Autodesk Inventor part; units mm, degrees
ref_plane "YZ Plane" through (0, 0, 0) normal (1, 0, 0) x (0, 1, 0)
ref_plane "XZ Plane" through (0, 0, 0) normal (0, 1, 0) x (-1, 0, 0)
ref_plane "XY Plane" through (0, 0, 0) normal (0, 0, 1) x (1, 0, 0)
sketch "Эскиз1" plane through (0, 0, 0) normal (0, 1, 0) x (-1, 0, 0)
  line L0 (0, 0) -> (60, 0)
  line L1 (60, 0) -> (60, -45)
  line L2 (60, -45) -> (0, -45)
  line L3 (0, -45) -> (0, 0)
  line L4 (0, -22.5) -> (0, 0)
  line L5 (0, 0) -> (0, -10)
  line L6 (0, -10) -> (35, -10)
  line L7 (35, -10) -> (35, -35)
  line L8 (35, -35) -> (0, -35)
  line L9 (35, -22.5) -> (45, -22.5)
  dimension "d0" = 60
  dimension "d1" = 45
  dimension "d3" = 10
  dimension "d4" = 35
  dimension "d5" = 25
  dimension "d6" = 10
extrude "Выдавливание1" add sketch "Эскиз1" along normal blind 10 contours L0 L1 L2 L3 L8 L7 L6
sketch "Эскиз3" plane through (0, 0, -35) normal (1, 0, 0) x (0, 0, -1)
  line L0 (10, 10) -> (-35, 10)
  line L1 (10, 10) -> (-35, 10)
  line L2 (-35, 10) -> (-35, -26)
  line L3 (-35, -26) -> (10, -26)
  line L4 (10, -26) -> (10, 10)
  point P0 (-35, 0)
  dimension "d13" = 45
  dimension "d14" = 36
extrude "Выдавливание3" add sketch "Эскиз3" along normal blind 5
sketch "Эскиз4" plane through (0, -26, -45) normal (0, -1, 0) x (1, 0, 0)
  line L0 (-60, 0) -> (0, 0)
  line L1 (0, 0) -> (0, 45)
  line L2 (0, 45) -> (-60, 45)
  line L3 (-60, 45) -> (-60, 0)
  line L4 (0, 35) -> (-35, 35)
  line L5 (-35, 10) -> (0, 10)
  line L6 (0, 10) -> (0, 35)
  line L7 (0, 35) -> (-35, 35)
  line L8 (-35, 35) -> (-35, 10)
extrude "Выдавливание4" add sketch "Эскиз4" against normal blind 10 contours L3 L2 L1 L4 L8 L5 L0
sketch "Эскиз5" plane through (0, 0, 0) normal (0, -1, 0) x (1, 0, 0)
  line L0 (-35, -10) -> (-35, -35)
  line L1 (-35, -22.5) -> (-45, -22.5)
  circle A0 centre (-45, -22.5) radius 5
  point P0 (0, 0)
  dimension "d19" = 10
  dimension "d20" = 10
extrude "Выдавливание5" cut sketch "Эскиз5" along normal blind 24 and the other way blind 6
sketch "Эскиз6" plane through (5, -26, -45) normal (0, -1, 0) x (1, 0, 0)
  line L0 (0, 0) -> (0, 45)
  line L1 (-65, 0) -> (0, 0)
  line L2 (0, 45) -> (-5, 45)
  line L3 (-5, 45) -> (-5, 0)
  line L4 (-5, 0) -> (0, 0)
  line L5 (0, 0) -> (0, 45)
extrude "Выдавливание6" add sketch "Эскиз6" along normal blind 50
sketch "Эскиз7" plane through (5, -76, -45) normal (0, -1, 0) x (1, 0, 0)
  line L0 (-65, 45) -> (0, 45)
  line L1 (0, 45) -> (-65, 45)
  line L2 (-65, 45) -> (-65, 0)
  line L3 (-65, 0) -> (0, 0)
  line L4 (0, 0) -> (0, 45)
  line L5 (-5, 10) -> (-5, 35)
  line L6 (-5, 22.5) -> (-15, 22.5)
  line L7 (-15, 22.5) -> (-17.5, 22.5)
  circle A0 centre (-17.5, 22.5) radius 2.5
  point P0 (-5, 45)
  dimension "d27" = 10
  dimension "d28" = 2.5
extrude "Выдавливание7" add sketch "Эскиз7" along normal blind 1
sketch "Эскиз8" plane through (0, 0, -35) normal (-1, 0, 0) x (0, 0, 1)
  line L0 (0, 0) -> (-10, 0)
  line L1 (-10, -16) -> (35, -16)
  line L2 (-10, 0) -> (-5, 0)
  line L3 (-5, 0) -> (-5, -16)
  line L4 (-5, -16) -> (-10, -16)
  line L5 (-10, -16) -> (-10, 0)
  line L6 (-10, 0) -> (35, 0)
  line L7 (35, -16) -> (30, -16)
  line L8 (30, -16) -> (30, 0)
  line L9 (30, 0) -> (35, 0)
  line L10 (35, 0) -> (35, -16)
  point P0 (25, -16)
  point P1 (-5, 0)
  dimension "d31" = 5
  dimension "d34" = 5
extrude "Выдавливание8" add sketch "Эскиз8" along normal blind 10 contours L3 L1 L5 L0 | L6 L10 L1 L8
properties part number "Стенка"
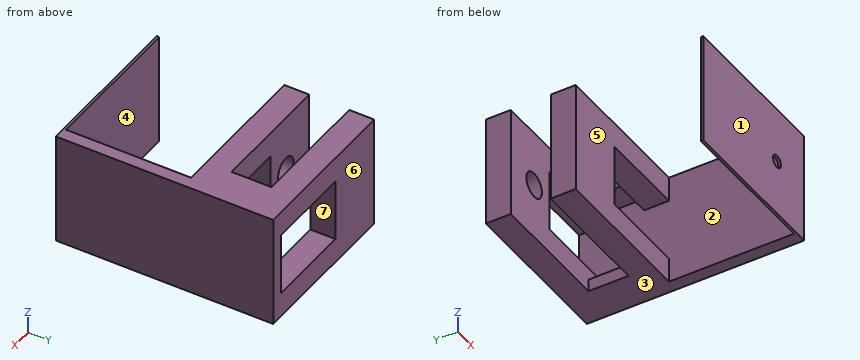
Design review of the part built by this model. Coordinates are the model's own, in mm. Face numbers are marked on the shaded views. A direction names the side the tool comes from. Give positions to 0.01 mm unless a question says otherwise; leave off trailing zeros. Order: outer loops, then holes, each group sorted by start corner. A loop starts at its lowest first (then second) coordinate and runs counter-clockwise, first axis right, second up. Notation, with made-up numbers: (-39.5, -37) - (-27.5, -37) arc R23 ccw to (-27.5, -24) - close; hole circle Ø6 at (-12.5, -38). An arc over 180 degrees is marked (long way). Use a Markdown table: item, result. Add a question column.
(1) Add section B-B on z = -22.5. Give the boundary of the cut face in (x, y), then the cut area to 3 significant figures.
(2) Add section D-D on z = -31.5. Give the boundary of the cut face in (x, y).
(3) Add section C-C on x = -12.5. Give the boundary of the cut face in (y, z).
(4) Mouldability with a two-part tool opening along Y and no side actions: class the marked faces 1, 2, 3 and 4 as +Y half, -Y half, draft (parallel to the pull), parting line (faces both ways), or undercut.
(5) Machinability: for the marked faces 5, 6 and 7, which of the approach directions +Z, -Z, +X, -X, +Y, -Y give a long, thin tool a straight path to every point of the face, cutting with its end or side? Answer none if there is none.
(6) Wall thickness on probe 1 along Y at (x, z) = (-49, -15.5); probe 2 along Z at (x, y) = (-8, -17); probe 3 along X at (y, z) = (-13.5, -18.5): over which ranges is each line inside the solid? List them lowest first. Write a range as [from, to].
(7) Clearance check with flat-ended pins moving along their axes: P1, Ø13.5, axis at x = -32, z = -24, coming from the +Y side; P2, Ø5.5, axis at y = -8.5, z = -1.5, coming from the -X side; P3, Ø4, axis at x = -12.5, z = -22.5, coming from the +Y side; P4, Ø5, axis at x = -15.5, z = -13, coming from the +Y side. State where each tip first meets the part, or that it passes through.
(8) Add section A-A on x = -27. Give the boundary of the cut face in (y, z), then the cut area to 3 significant figures.
Report:
| question | item | result |
|---|---|---|
| 1 | outline | (-60, -77) - (-15, -77) - (-15, -76) - (-60, -76) - close; (-60, -26) - (-35, -26) - (-35, -16) - (-40, -16) - (-40, -24) - (-50, -24) - (-50, -16) - (-60, -16) - close; (-60, 0) - (-50, 0) - (-50, 6) - (-40, 6) - (-40, 0) - (-35, 0) - (-35, 10) - (-60, 10) - close; (-10, -77) - (5, -77) - (5, 10) - (0, 10) - (0, -76) - (-10, -76) - close |
| 1 | area | 850 mm² |
| 2 | outline | (-60, -77) - (5, -77) - (5, 10) - (0, 10) - (0, -76) - (-60, -76) - close; (-60, -26) - (-35, -26) - (-35, -16) - (-60, -16) - close; (-60, 0) - (-35, 0) - (-35, 10) - (-60, 10) - close |
| 3 | outline | (-77, -45) - (-76, -45) - (-76, -25) - (-77, -25) - close; (-77, -20) - (-76, -20) - (-76, 0) - (-77, 0) - close; (-26, -45) - (-16, -45) - (-16, -35) - (-26, -35) - close; (-26, -10) - (-16, -10) - (-16, 0) - (-26, 0) - close; (0, -45) - (10, -45) - (10, -35) - (0, -35) - close; (0, -10) - (10, -10) - (10, 0) - (0, 0) - close |
| 4 | face 1 | -Y half |
| 4 | face 2 | undercut |
| 4 | face 3 | draft |
| 4 | face 4 | undercut |
| 5 | face 5 | +Z, -Z, -X |
| 5 | face 6 | +Z, -Z, +X, -X, +Y |
| 5 | face 7 | +Y |
| 6 | probe 1 | y = [-77, -76], [-26, -16], [0, 10] |
| 6 | probe 2 | z = [-45, -35], [-10, 0] |
| 6 | probe 3 | x = [0, 5] |
| 7 | P1 | stops at y = 10 |
| 7 | P2 | stops at x = -10 |
| 7 | P3 | passes through |
| 7 | P4 | stops at y = -76 |
| 8 | outline | (-77, -45) - (-76, -45) - (-76, 0) - (-77, 0) - close; (-26, -45) - (-16, -45) - (-16, -35) - (-26, -35) - close; (-26, -10) - (-16, -10) - (-16, 0) - (-26, 0) - close; (0, -45) - (10, -45) - (10, -35) - (0, -35) - close; (0, -10) - (10, -10) - (10, 0) - (0, 0) - close |
| 8 | area | 445 mm² |
